```python
from build123d import *

# Parameters (mm, degrees)
SKETCH1_W           = 65
SKETCH1_H           = 102
SKETCH1_R           = 2.5
SKETCH1_R_2         = 2
BOSS_EXTRUDE1_DEPTH = 3.175
CHAMFER1_SIZE       = 5


with BuildPart() as part:
    # Sketch1 → Boss-Extrude1 (new body)
    with BuildSketch(Plane.XY):
        Rectangle(SKETCH1_W, SKETCH1_H)
        with Locations((24.5, 36)):
            Circle(SKETCH1_R, mode=Mode.SUBTRACT)
        with Locations((-24.5, 36)):
            Circle(SKETCH1_R, mode=Mode.SUBTRACT)
        with Locations((26.5, 0)):
            Circle(SKETCH1_R_2, mode=Mode.SUBTRACT)
        with Locations(Location((-26.5, 0, 0), (0, 0, 180))):
            Circle(SKETCH1_R_2, mode=Mode.SUBTRACT)
        with Locations((-26.5, -37)):
            Circle(SKETCH1_R_2, mode=Mode.SUBTRACT)
        with Locations(Location((26.5, -37, 0), (0, 0, 180))):
            Circle(SKETCH1_R_2, mode=Mode.SUBTRACT)
    extrude(amount=BOSS_EXTRUDE1_DEPTH)

    # Chamfer1
    chamfer1_edges = [part.edges().sort_by_distance(p)[0] for p in [
        (32.5, -51, 1.5875),
        (-32.5, -51, 1.5875),
        (-32.5, 51, 1.5875),
        (32.5, 51, 1.5875),
    ]]
    chamfer(chamfer1_edges, length=CHAMFER1_SIZE)


solid = part.part
```
Model file for the job. Use its own axes, mm. Round coordinates to 2 decimals unless told otherwise and drop trailing zeros. Order: outer loops, then holes, each group sorted by start corner. A loop starts at its lowest first (then second) coordinate and runs counter-clockwise, first axis right, second up. Notation, with made-up numbers: (-26, 72.5) -> (-21, 72.5) arc R34 ccw to (-21, 108.5) -> close; hole circle Ø9 at (-35, -18.5). An arc over 180 degrees is marked (long way). Use one line per item in the form item = value.
Item 1: Pull direction Y, two halves, no side cores. Call faces 1 (the face through (0, 1, 0)), 2 (the face through (0, 51, 2)), 3 (the face through (-25.04, 33.56, 1.57)): released by +Y, released by -Y, zero draft, split by the parting line, or undercut.
Returned:
face_1 = zero draft
face_2 = released by +Y
face_3 = undercut
Item 2: Cut at C-C, the plane x = 26. Write the cut outline in (y, z) (1 decimal).
Returned:
outline = (-51, 0) -> (-38.9, 0) -> (-38.9, 3.2) -> (-51, 3.2) -> close; (-35.1, 0) -> (-1.9, 0) -> (-1.9, 3.2) -> (-35.1, 3.2) -> close; (1.9, 0) -> (34, 0) -> (34, 3.2) -> (1.9, 3.2) -> close; (38, 0) -> (51, 0) -> (51, 3.2) -> (38, 3.2) -> close
Item 3: Cut at D-D, the plane y = 36. Write the cut outline in (x, z) (3 decimals).
Returned:
outline = (-32.5, 0) -> (-27, 0) -> (-27, 3.175) -> (-32.5, 3.175) -> close; (-22, 0) -> (22, 0) -> (22, 3.175) -> (-22, 3.175) -> close; (27, 0) -> (32.5, 0) -> (32.5, 3.175) -> (27, 3.175) -> close
Item 4: Cut at B-B, the plane z = 1.35. Write the cut outline in (x, y).
Returned:
outline = (-32.5, -46) -> (-27.5, -51) -> (27.5, -51) -> (32.5, -46) -> (32.5, 46) -> (27.5, 51) -> (-27.5, 51) -> (-32.5, 46) -> close; hole circle Ø4 at (-26.5, -37); hole circle Ø4 at (-26.5, 0); hole circle Ø5 at (-24.5, 36); hole circle Ø5 at (24.5, 36); hole circle Ø4 at (26.5, -37); hole circle Ø4 at (26.5, 0)
Item 5: Flat gauge pin, fed straight in: pin 1 Ø2.5 at (x, y) = (26.5, 0) entering from -Z (3 decimals). Where does the tip first touch, or does it go through?
Returned:
pin_1 = through
Item 6: Drill centre lines: line 1 (Y direction, x = 26.5, z = 1.35); line 2 (X direction, y = 35.5, z = 1.5); line 3 (Y direction, x = -23, z = 2.35). Where is each one in solid material? Low to high.
Returned:
line_1 = -51 to -39, -35 to -2, 2 to 34.5, 37.5 to 51
line_2 = -32.5 to -26.95, -22.05 to 22.05, 26.95 to 32.5
line_3 = -51 to 34, 38 to 51
Item 7: Cut at A-A, the plane y = -37. Write the cut outline in (x, z) (3 decimals), and give its area (3 significant figures).
Returned:
outline = (-32.5, 0) -> (-28.5, 0) -> (-28.5, 3.175) -> (-32.5, 3.175) -> close; (-24.5, 0) -> (24.5, 0) -> (24.5, 3.175) -> (-24.5, 3.175) -> close; (28.5, 0) -> (32.5, 0) -> (32.5, 3.175) -> (28.5, 3.175) -> close
area = 181 mm^2
